Verification items for the finished model (mm, model axes). A direction names the side the tool comes from. Give positions to 0.01 mm unless a question says otherwise; leave off trailing zeros. Write each loop counter-clockwise with the first axis right and the second up, starting at its lowest first coordinate (ties: lowest second). Pieces come first, ordered by that corner, then holes. Notation, with made-up numbers: (18, -16) - (37, -16) arc R23 cw to (37, -5) - close; hole circle Ø3 at (-34.5, 59). An arc over 180 degrees is marked (long way). Put each result on its own line as item: value.
from build123d import *

# Parameters (mm, degrees)
SKETCH1_R           = 5
SKETCH1_R_2         = 1.5
BOSS_EXTRUDE1_DEPTH = 6
BOSS_EXTRUDE2_DEPTH = 6
CUT_EXTRUDE2_DEPTH  = 7
CUT_EXTRUDE3_DEPTH  = 10


with BuildPart() as part:
    # Sketch1 → Boss-Extrude1 (new body)
    with BuildSketch(Plane(origin=(0, 0, 0), x_dir=(0, 0, -1), z_dir=(1, 0, 0))):
        with Locations((5, 5)):
            Circle(SKETCH1_R)
        with Locations((5, 5)):
            Circle(SKETCH1_R_2, mode=Mode.SUBTRACT)
        with BuildLine():
            ThreePointArc((10, 5), (8.535533906, 1.464466094), (5, 0))
            Line((5, 0), (27, 0))
            ThreePointArc((27, 0), (22, 5), (27, 10))
            Line((27, 10), (5, 10))
            ThreePointArc((5, 10), (8.535533906, 8.535533906), (10, 5))
        make_face()
        with Locations((27, 5)):
            Circle(SKETCH1_R)
        with Locations((27, 5)):
            Circle(SKETCH1_R_2, mode=Mode.SUBTRACT)
    extrude(amount=BOSS_EXTRUDE1_DEPTH)

    # Sketch2 → Boss-Extrude2 (add)
    with BuildSketch(Plane(origin=(6, 0, 0), x_dir=(0, 0, -1), z_dir=(1, 0, 0))):
        with BuildLine():
            ThreePointArc((27, 10), (29.694507461, 9.21184396), (31.53953799, 7.095851816))
            Line((31.53953799, 7.095851816), (31.610157793, 7.262674791))
            Line((31.610157793, 7.262674791), (44.585599673, 12.519851602))
            Line((44.585599673, 12.519851602), (51.097249205, 9.763328363))
            Line((51.097249205, 9.763328363), (60.365421977, 13.518454657))
            Line((60.365421977, 13.518454657), (56.610295683, 22.786627428))
            Line((56.610295683, 22.786627428), (25.051124858, 10))
            Line((25.051124858, 10), (27, 10))
        make_face()
        Polygon((60.365421977, 13.518454657), (51.097249205, 9.763328363), (51.333822162, 9.179433479), (60.601994933, 12.934559772), align=None)
    extrude(amount=-BOSS_EXTRUDE2_DEPTH)

    # Sketch4 → Cut-Extrude2 (cut, through all)
    with BuildSketch(Plane(origin=(6, 0, 0), x_dir=(0, 0, -1), z_dir=(1, 0, 0))):
        Polygon((56.610295683, 22.786627428), (51.684261855, 20.790777803), (58.606145308, 17.8605936), align=None)
    extrude(amount=-CUT_EXTRUDE2_DEPTH, mode=Mode.SUBTRACT)

    # Sketch5 → Cut-Extrude3 (cut)
    with BuildSketch(Plane(origin=(6, 0, 0), x_dir=(0, 0, -1), z_dir=(1, 0, 0))):
        with BuildLine():
            ThreePointArc((27, 0), (31.21184396, 2.305492539), (31.53953799, 7.095851816))
            Line((31.53953799, 7.095851816), (29.583779735, 2.664986829))
            Line((29.583779735, 2.664986829), (25.539598719, 0))
            Line((25.539598719, 0), (27, 0))
        make_face()
        Polygon((52.260639439, 9.554946108), (51.097249205, 9.763328363), (51.333822162, 9.179433479), align=None)
        Polygon((52.95088376, 10.514353622), (52.260639439, 9.554946108), (54.114273993, 10.305971367), align=None)
        Polygon((54.804518314, 11.265378881), (54.114273993, 10.305971367), (55.967908548, 11.056996626), align=None)
        Polygon((56.658152868, 12.01640414), (55.967908548, 11.056996626), (57.821543102, 11.808021884), align=None)
        Polygon((58.511787422, 12.767429398), (57.821543102, 11.808021884), (59.675177656, 12.559047143), align=None)
        Polygon((60.365421977, 13.518454657), (59.675177656, 12.559047143), (60.601994933, 12.934559772), align=None)
    extrude(amount=-CUT_EXTRUDE3_DEPTH, mode=Mode.SUBTRACT)


solid = part.part
Q1. Scan lines: line 1 along Y through (x, z) = (2, -20); line 2 along Y through (x, z) = (3.45, -5); line 3 along Y through (x, z) = (3.5, -27). Record each from-to range of solid material in increasing order.
Answers follow:
line 1: y = 0 to 10
line 2: y = 0 to 3.5, 6.5 to 10
line 3: y = 0.96 to 3.5, 6.5 to 10.79
Q2. Go/stop test with flat-tipped pins: pin 1 Ø1 at (y, z) = (10, -22.5) entering from -X; pin 2 Ø1.5 at (x, z) = (3.5, -44.5) entering from -Y; pin 3 Ø2.5 at (y, z) = (5, -27) entering from -X; pin 4 Ø1 at (x, z) = (3.5, -8) entering from +Y. Record where each tip stops, or that it passes through.
Answers follow:
pin 1: stops at x = 0
pin 2: stops at y = 12.18
pin 3: passes through
pin 4: stops at y = 10
Q3. Section check D-D, the plane z = -11. Record the cut outline in (x, y).
Answers follow:
outline: (0, 0) - (6, 0) - (6, 10) - (0, 10) - close
Q4. Section check B-B, the plane z = -27. Record the cut outline in (x, y), plus the area to 3 significant figures.
Answers follow:
outline: (0, 0.96) - (6, 0.96) - (6, 3.5) - (0, 3.5) - close; (0, 6.5) - (6, 6.5) - (6, 10.79) - (0, 10.79) - close
area: 41.0 mm2
Q5. Set-up check for faces 1 (the face through (3.042, 9.854, -38.007)), 2 (the face through (3, 0, -15)), 3 (the face through (3, 10, -15)): record each of +Z, -Z, +X, -X, +Y, -Y from which the full face is reachable in a straight line by a thin tool's end or side.
Answers follow:
face 1: +X, -X, -Y
face 2: +Z, -Z, +X, -X, -Y
face 3: +Z, +X, -X, +Y
Q6. Section check C-C, the plane y = 5. Record the cut outline in (x, z), plus the area to 3 significant figures.
Answers follow:
outline: (0, -30.61) - (6, -30.61) - (6, -28.5) - (0, -28.5) - close; (0, -25.5) - (6, -25.5) - (6, -6.5) - (0, -6.5) - close; (0, -3.5) - (6, -3.5) - (6, 0) - (0, 0) - close
area: 148 mm2
Q7. Section check A-A, the plane x = 3.75. Record the cut outline in (y, z).
Answers follow:
outline: (0, -25.54) - (2.66, -29.58) - (7.1, -31.54) - (7.26, -31.61) - (12.52, -44.59) - (9.76, -51.1) - (9.55, -52.26) - (10.51, -52.95) - (10.31, -54.11) - (11.27, -54.8) - (11.06, -55.97) - (12.02, -56.66) - (11.81, -57.82) - (12.77, -58.51) - (12.56, -59.68) - (13.52, -60.37) - (17.86, -58.61) - (20.79, -51.68) - (10, -25.05) - (10, -5) arc R5 ccw to (0, -5) - close; hole circle Ø3 at (5, -27); hole circle Ø3 at (5, -5)
Q8. Release check for a two-part mould opening along Y. For faces 4 (the face through (3.04, 15.47, -38.55)), 5 (the face through (3.04, 1.35, -27.59)), 6 (the face through (2.96, 5.07, -25.5)), 7 (the face through (2.958, 4.425, -6.386)) record: released by +Y, released by -Y, zero draft, split by the parting line, or undercut.
Answers follow:
face 4: released by +Y
face 5: released by -Y
face 6: undercut
face 7: undercut
